Geometry check sheet. Reference: the model listing, model coordinates, mm. Face numbers are marked on the shaded views. Give positions to 0.01 mm unless a question says otherwise; leave off trailing zeros. Write each loop counter-clockwise with the first axis right and the second up, starting at its lowest first coordinate (ties: lowest second). Pieces come first, ordered by that corner, then holes.
(1) Cross-section at D-D (y = -41.5). Record the boundary of the cut face in (x, z), and give its area (3 significant figures).
(2) Cross-section at C-C (z = 37). Record the boundary of the cut face in (x, y), and give its area (3 significant figures).
(3) Mould release check, pull along Y, two halves, no side actions. Record for the marked faces 1, 2 and 3: +Y half, -Y half, draft (parallel to the pull), parting line (faces both ways), or undercut.
(4) Depth check by flat-ended pin: P1, Ø6, axis at x = 62.5, y = 8, coming from the +Z side; P2, Ø2, axis at x = 139, z = 24.5, coming from the -Y side; P3, Ø12, axis at x = 83, z = 41, coming from the -Y side. Enter the tip coordinate at first touch or a pass-through.
(5) Cross-section at A-A (z = 20). Record the boundary of the cut face in (x, y).
(6) Thickness scan on line 1 along Y through (x, z) = (14, 28); line 2 along Y through (x, z) = (63, 29); line 3 along Z through (x, y) = (60, 29.5). Record the ranges inside material, lowest first.
(7) Cross-section at B-B (x = 114). Record the boundary of the cut face in (y, z), and give its area (3 significant figures).
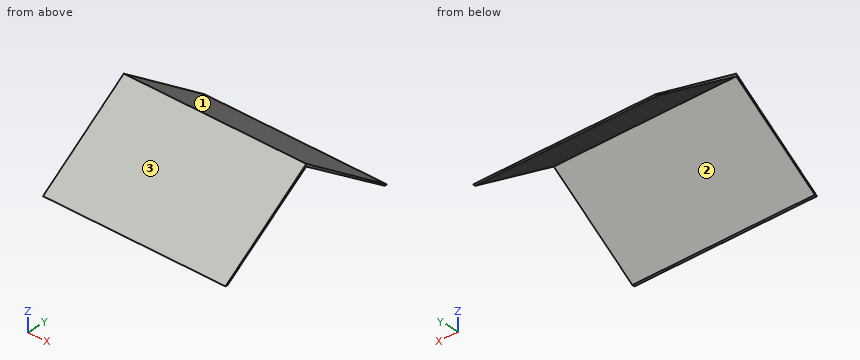
```python
from build123d import *

# Parameters (mm, degrees)
F1_DEPTH = 190.5


with BuildPart() as f1:
    # F0 (on Right) → F1 (new body)
    with BuildSketch(Plane.YZ):
        Polygon((0, 67.456241), (-95.25, 0), (-92.71, 0), (0, 64.916241), align=None)
        Polygon((95.25, 0), (0, 67.456241), (0, 64.916241), (92.71, 0), align=None)
    extrude(amount=F1_DEPTH)


solid = f1.part
```
Reply:
1. outline: (0, 35.86) - (190.5, 35.86) - (190.5, 38.07) - (0, 38.07) - close
1. area: 421 mm2
2. outline: (0, -43.01) - (190.5, -43.01) - (190.5, -39.87) - (0, -39.87) - close; (0, 39.87) - (190.5, 39.87) - (190.5, 43.01) - (0, 43.01) - close
2. area: 1,200 mm2
3. face 1: +Y half
3. face 2: undercut
3. face 3: -Y half
4. P1: stops at z = 63.92
4. P2: stops at y = -62.07
4. P3: stops at y = -45.83
5. outline: (0, -67.01) - (190.5, -67.01) - (190.5, -64.15) - (0, -64.15) - close; (0, 64.15) - (190.5, 64.15) - (190.5, 67.01) - (0, 67.01) - close
6. line 1: y = -55.71 to -52.72, 52.72 to 55.71
6. line 2: y = -54.3 to -51.29, 51.29 to 54.3
6. line 3: z = 44.26 to 46.56
7. outline: (-95.25, 0) - (-92.71, 0) - (0, 64.92) - (92.71, 0) - (95.25, 0) - (0, 67.46) - close
7. area: 407 mm2
